Can you work these out from the model? Positions are in its coordinate system, mm. Face numbers are marked on the shaded views. A direction names the side the tool comes from. Give positions to 0.01 mm unless a question says otherwise; leave off trailing zeros. Order: outer loops, then holes, each group sorted by start corner. A loop starts at its lowest first (then second) coordinate and runs counter-clockwise, first axis right, second up. Notation, with made-up numbers: (37.5, 83) - (87.5, 83) arc R18 ccw to (87.5, 99) - close; hole circle Ø9 at (-3.5, -39.75). An arc over 180 degrees is marked (long way). Use one line per item in the form item = value. Start each with the question number.
1) Suppose I cut it at A-A, the plane y = 12.75. Write out the boundary of the cut face in (x, z).
2) We'd pull the mould along Z, two halves only. Please class the marked faces 3, 4, 5 and 6: released by +Z, released by -Z, zero draft, split by the parting line, or undercut.
3) Please list where these lines run through material, in increasing order: probe 1 along Z at (x, y) = (8.75, 19); probe 2 along Y at (x, z) = (6.75, -17.5); probe 3 along X at (y, z) = (14, -34.5).
4) Suppose I cut it at C-C, the plane z = -43.5. Write out the boundary of the cut face in (x, y).
5) Which directions (+Z, -Z, +X, -X, +Y, -Y) give clear straight access to the entire face, cutting with the end or side of a thin tool? Please do the marked faces 1 and 2.
6) For pin 1 (2 mm diameter, centred on y = 18.5, z = -30, fed in from +X); pin 2 (2 mm diameter, centred on x = 5, y = 6.5, fed in from -Z), each with a flat end and sliding along its axis, tell me the tip position at first contact or that it passes through.
7) Suppose I cut it at B-B, the plane x = 8.25. Write out the boundary of the cut face in (y, z).
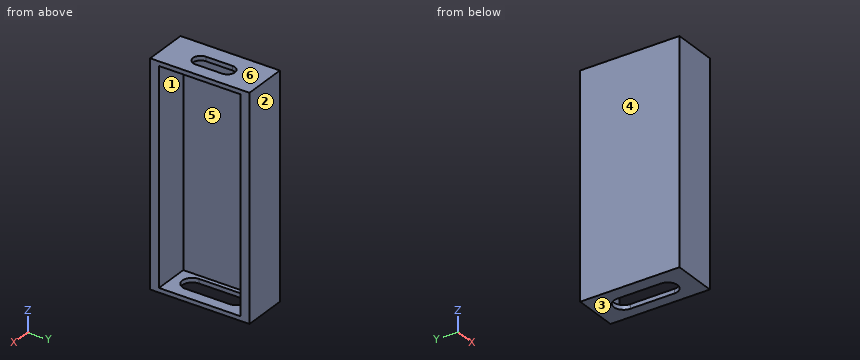
```python
from build123d import *

# Parameters (mm, degrees)
SKETCH2_W           = 50
SKETCH2_H           = 22.5
BOSS_EXTRUDE1_DEPTH = 10
USBC_DEPTH          = 10
POGO_DEPTH          = 10
SKETCH6_W           = 48
SKETCH6_H           = 18.5
CUT_EXTRUDE3_DEPTH  = 8


with BuildPart() as part:
    # Sketch2 → Boss-Extrude1 (new body)
    with BuildSketch(Plane(origin=(0, 0, 0), x_dir=(0, 0, -1), z_dir=(1, 0, 0))):
        with Locations((25, 11.25)):
            Rectangle(SKETCH2_W, SKETCH2_H)
    extrude(amount=BOSS_EXTRUDE1_DEPTH)

    # Sketch4 → USBC (cut)
    with BuildSketch(Plane.XY):
        with BuildLine():
            Line((7.05, 14.275), (7.05, 8.225))
            ThreePointArc((7.05, 8.225), (5.325, 6.5), (3.6, 8.225))
            Line((3.6, 8.225), (3.6, 14.275))
            ThreePointArc((3.6, 14.275), (5.325, 16), (7.05, 14.275))
        make_face()
    extrude(amount=-USBC_DEPTH, mode=Mode.SUBTRACT)

    # Sketch5 → POGO (cut)
    with BuildSketch(Plane(origin=(0, 0, -50), x_dir=(-1, 0, 0), z_dir=(0, 0, -1))):
        with BuildLine():
            Line((-3, 16.25), (-3, 6.25))
            ThreePointArc((-3, 6.25), (-5.225, 4.025), (-7.45, 6.25))
            Line((-7.45, 6.25), (-7.45, 16.25))
            ThreePointArc((-7.45, 16.25), (-5.225, 18.475), (-3, 16.25))
        make_face()
    extrude(amount=-POGO_DEPTH, mode=Mode.SUBTRACT)

    # Sketch6 → Cut-Extrude3 (cut)
    with BuildSketch(Plane(origin=(10, 0, 0), x_dir=(0, 0, -1), z_dir=(1, 0, 0))):
        with Locations((25, 11.25)):
            Rectangle(SKETCH6_W, SKETCH6_H)
    extrude(amount=-CUT_EXTRUDE3_DEPTH, mode=Mode.SUBTRACT)


solid = part.part
```
Result sheet:
q1.outline = (0, -50) - (3, -50) - (3, -49) - (2, -49) - (2, -1) - (3.6, -1) - (3.6, 0) - (0, 0) - close; (7.05, -1) - (10, -1) - (10, 0) - (7.05, 0) - close; (7.45, -50) - (10, -50) - (10, -49) - (7.45, -49) - close
q2.face_3 = released by -Z
q2.face_4 = zero draft
q2.face_5 = undercut
q2.face_6 = released by +Z
q3.probe_1 = -50 to -49, -1 to 0
q3.probe_2 = 0 to 2, 20.5 to 22.5
q3.probe_3 = 0 to 2
q4.outline = (0, 0) - (10, 0) - (10, 2) - (2, 2) - (2, 20.5) - (10, 20.5) - (10, 22.5) - (0, 22.5) - close
q5.face_1 = +X
q5.face_2 = +Z, -Z, +X, -X, +Y
q6.pin_1 = 2
q6.pin_2 = -1
q7.outline = (0, -50) - (22.5, -50) - (22.5, 0) - (0, 0) - close; hole (2, -49) - (20.5, -49) - (20.5, -1) - (2, -1) - close
